from build123d import *

# Parameters (mm, degrees)
BOSS_EXTRUDE1_DEPTH = 10
CHAMFER1_SIZE       = 6
CHAMFER1_SIZE2      = 16
CHAMFER2_SIZE       = 16
CHAMFER2_SIZE2      = 6
SKETCH2_W           = 10
SKETCH2_H           = 10
CUT_EXTRUDE1_DEPTH  = 10
BOSS_EXTRUDE2_DEPTH = 7
SKETCH4_R           = 5
SKETCH4_R_2         = 4.7
CUT_EXTRUDE2_DEPTH  = 3
SKETCH5_R           = 2.15
CUT_EXTRUDE3_DEPTH  = 11
SKETCH6_R           = 4
CUT_EXTRUDE4_DEPTH  = 6
SKETCH7_R           = 2.4
BOSS_EXTRUDE3_DEPTH = 4.6
SKETCH8_R           = 1.65
CUT_EXTRUDE5_DEPTH  = 10
BOSS_EXTRUDE4_DEPTH = 66


with BuildPart() as part:
    # Sketch1 → Boss-Extrude1 (new body)
    with BuildSketch(Plane(origin=(0, 0, 0), x_dir=(1, 0, 0), z_dir=(0, 1, 0))):
        Polygon((0, 0), (0, -45), (86, -45), (86, 31), (33, 31), (14, 0), align=None)
    extrude(amount=BOSS_EXTRUDE1_DEPTH)

    # Chamfer1
    chamfer1_edges = [part.edges().sort_by_distance(p)[0] for p in [
        (86, 5, 45),
    ]]
    chamfer1_side = [part.faces().sort_by_distance(p)[0] for p in [
        (43, 5, 45),
    ]]
    chamfer(chamfer1_edges, length=CHAMFER1_SIZE, length2=CHAMFER1_SIZE2, reference=chamfer1_side[0])

    # Chamfer2
    chamfer2_edges = [part.edges().sort_by_distance(p)[0] for p in [
        (0, 5, 45),
    ]]
    chamfer2_side = [part.faces().sort_by_distance(p)[0] for p in [
        (0, 5, 22.5),
    ]]
    chamfer(chamfer2_edges, length=CHAMFER2_SIZE, length2=CHAMFER2_SIZE2, reference=chamfer2_side[0])

    # Sketch2 → Cut-Extrude1 (cut)
    with BuildSketch(Plane(origin=(0, 10, 0), x_dir=(1, 0, 0), z_dir=(0, 1, 0))):
        with Locations((81, 26)):
            Rectangle(SKETCH2_W, SKETCH2_H)
    extrude(amount=-CUT_EXTRUDE1_DEPTH, mode=Mode.SUBTRACT)

    # Sketch3 → Boss-Extrude2 (add)
    with BuildSketch(Plane.XZ):
        with BuildLine():
            Line((44.7, 2.297872822), (44.7, 11.702127178))
            ThreePointArc((44.7, 11.702127178), (43, 12), (41.3, 11.702127178))
            Line((41.3, 11.702127178), (41.3, 2.297872822))
            ThreePointArc((41.3, 2.297872822), (43, 2), (44.7, 2.297872822))
        make_face()
    extrude(amount=BOSS_EXTRUDE2_DEPTH)

    # Sketch4 → Cut-Extrude2 (cut)
    with BuildSketch(Plane.XZ.offset(7)):
        with Locations((43, 7)):
            Circle(SKETCH4_R)
        with Locations((43, 7)):
            Circle(SKETCH4_R_2, mode=Mode.SUBTRACT)
    extrude(amount=-CUT_EXTRUDE2_DEPTH, mode=Mode.SUBTRACT)

    # Sketch5 → Cut-Extrude3 (cut, through all)
    with BuildSketch(Plane.XZ):
        with Locations((74.5, 35.5)):
            Circle(SKETCH5_R)
        with Locations((11, 35.5)):
            Circle(SKETCH5_R)
        with Locations((74.5, -5.8)):
            Circle(SKETCH5_R)
    extrude(amount=-CUT_EXTRUDE3_DEPTH, mode=Mode.SUBTRACT)

    # Sketch6 → Cut-Extrude4 (cut)
    with BuildSketch(Plane(origin=(0, 10, 0), x_dir=(1, 0, 0), z_dir=(0, 1, 0))):
        with Locations((74.5, 5.8)):
            Circle(SKETCH6_R)
        with Locations((74.5, -35.5)):
            Circle(SKETCH6_R)
        with Locations((11, -35.5)):
            Circle(SKETCH6_R)
    extrude(amount=-CUT_EXTRUDE4_DEPTH, mode=Mode.SUBTRACT)

    # Sketch7 → Boss-Extrude3 (add)
    with BuildSketch(Plane.XZ):
        with Locations((61.4, 7)):
            Circle(SKETCH7_R)
        with Locations((24.6, 7)):
            Circle(SKETCH7_R)
    extrude(amount=BOSS_EXTRUDE3_DEPTH)

    # Sketch8 → Cut-Extrude5 (cut)
    with BuildSketch(Plane(origin=(0, 0, -31), x_dir=(-1, 0, 0), z_dir=(0, 0, -1))):
        with Locations((-43, 5)):
            Circle(SKETCH8_R)
    extrude(amount=-CUT_EXTRUDE5_DEPTH, mode=Mode.SUBTRACT)

    # Sketch10 → Boss-Extrude4 (add)
    with BuildSketch(Plane(origin=(0, 10, 0), x_dir=(1, 0, 0), z_dir=(0, 1, 0))):
        with BuildLine():
            Line((15, -60), (72, -60))
            ThreePointArc((72, -60), (80.485281374, -56.485281374), (84, -48))
            Line((84, -48), (84, -26))
            Line((84, -26), (8.731847537, -26))
            Line((8.731847537, -26), (8.731847537, 15))
            Line((8.731847537, 15), (7.231847537, 15))
            Line((7.231847537, 15), (3, -9))
            Line((3, -9), (3, -48))
            ThreePointArc((3, -48), (6.514718626, -56.485281374), (15, -60))
        make_face()
    extrude(amount=BOSS_EXTRUDE4_DEPTH)


solid = part.part
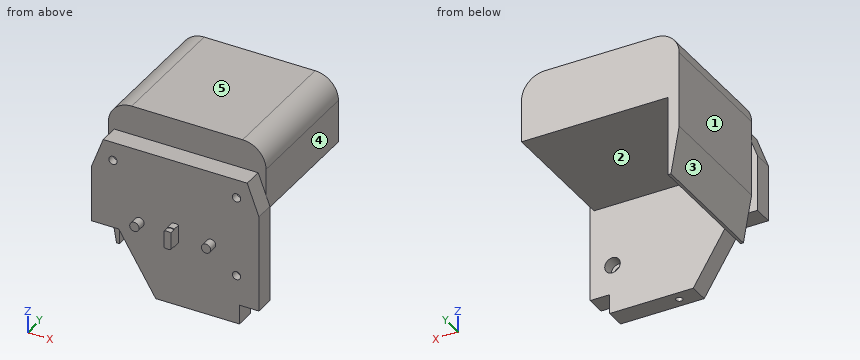
Source: CAD feature listing. Evaluate the final solid. Frame: model axes, mm. Face numbers are marked on the shaded views. A direction names the side the tool comes from. Coordinates: 2 decimals unless noted, no trailing zeros. Loops run counter-clockwise (first coordinate to the right, second up) from the corner with the lowest first, then second, coordinate; pieces in that order, holes last. Notation, with made-up numbers: M -32.75,-36.5 L 6.25,-36.5 A35 ccw 6.25,0.5 Z; hole C 72,14.25 d1. An arc over 180 degrees is marked long. Answer in a Markdown table with one row per item.
Q1. Section C-C on x = 74.5. Return the cut outline in (y, z).
Answers below:
| item | result |
|---|---|
| outline | M 0,-31 L 10,-31 L 10,-9.8 L 4,-9.8 L 4,-7.95 L 0,-7.95 Z; M 0,-3.65 L 4,-3.65 L 4,-1.8 L 10,-1.8 L 10,26 L 76,26 L 76,59.74 L 10,59.74 L 10,45 L 0,45 L 0,37.65 L 4,37.65 L 4,39.5 L 10,39.5 L 10,31.5 L 4,31.5 L 4,33.35 L 0,33.35 Z |
Q2. First-contact query: pin 1 (8 mm diameter, centred on x = 59, z = -12, fed in from -Y); pin 2 (2 mm diameter, centred on y = 65, z = 18, fed in from +X); pin 3 (5 mm diameter, centred on y = 7.5, z = -25.5, fed in from +X); pin 4 (11 mm diameter, centred on x = 44.5, y = 6.5, fed in from +Z). Flat tips, straight axial feed; report the tip coordinate or a pass-through.
Answers below:
| item | result |
|---|---|
| pin 1 | stops at y = 0 |
| pin 2 | stops at x = 8.73 |
| pin 3 | stops at x = 76 |
| pin 4 | stops at z = 60 |
Q3. Set-up query: the marked faces 1, 2, 3, 4 and 5. Return all of +Z, -Z, +X, -X, +Y, -Y with unobstructed straight access to the full face (end or side cutting, diameter ignored); none if empty.
Answers below:
| item | result |
|---|---|
| face 1 | +Z, -Z, -X, +Y |
| face 2 | -Z, +X, +Y |
| face 3 | -Z, -X, +Y |
| face 4 | +Z, -Z, +X, +Y |
| face 5 | +Z, +X, -X, +Y, -Y |
Q4. Section D-D on z = 7. Return the cut outline in (x, y), plus the area to 3 significant figures.
Answers below:
| item | result |
|---|---|
| outline | M 0,0 L 22.2,0 L 22.2,-4.6 L 27,-4.6 L 27,0 L 41.3,0 L 41.3,-7 L 44.7,-7 L 44.7,0 L 59,0 L 59,-4.6 L 63.8,-4.6 L 63.8,0 L 86,0 L 86,10 L 8.73,10 L 8.73,76 L 3.35,76 L 3.35,10 L 0,10 Z |
| area | 1,280 mm^2 |
Q5. Ray query, probe 1 along X at (y, z) = (8, 35); probe 2 along Z at (x, y) = (74, 8); probe 3 along X at (y, z) = (1, 35). Return the intervals inside material, ascending. Write a range as from..to.
Answers below:
| item | result |
|---|---|
| probe 1 | x = 2.25..7.03, 14.97..70.53, 78.47..83.75 |
| probe 2 | z = -31..-9.77, -1.83..31.53, 39.47..45 |
| probe 3 | x = 2.25..8.91, 13.09..72.41, 76.59..83.75 |
Q6. Section A-A on x = 61.4. Return the cut outline in (y, z), plus the area to 3 significant figures.
Answers below:
| item | result |
|---|---|
| outline | M -4.6,4.6 L 0,4.6 L 0,-31 L 10,-31 L 10,26 L 76,26 L 76,60 L 10,60 L 10,45 L 0,45 L 0,9.4 L -4.6,9.4 Z |
| area | 3,030 mm^2 |
Q7. Section B-B on y = 60. Return the cut outline in (x, z), plus the area to 3 significant figures.
Answers below:
| item | result |
|---|---|
| outline | M 3,9 L 7.23,-15 L 8.73,-15 L 8.73,26 L 84,26 L 84,48 A12 ccw 72,60 L 15,60 A12 ccw 3,48 Z |
| area | 2,880 mm^2 |
